Here's the drawing with two shaded views (mm, measured from the low corner). I have some questions. Round coordinates to 2 decimals unless told otherwise and drop trailing zeros. Loops run counter-clockwise (first coordinate to the right, second up) from the corner with the lowest first, then second, coordinate; pieces in that order, holes last. Notation, with made-up numbers: (7.5, 19) -> (37.5, 19) arc R24 ccw to (37.5, 58) -> close; hole circle Ø1 at (44.5, -14.75). An arc over 180 degrees is marked (long way). Write item = value, one per line.
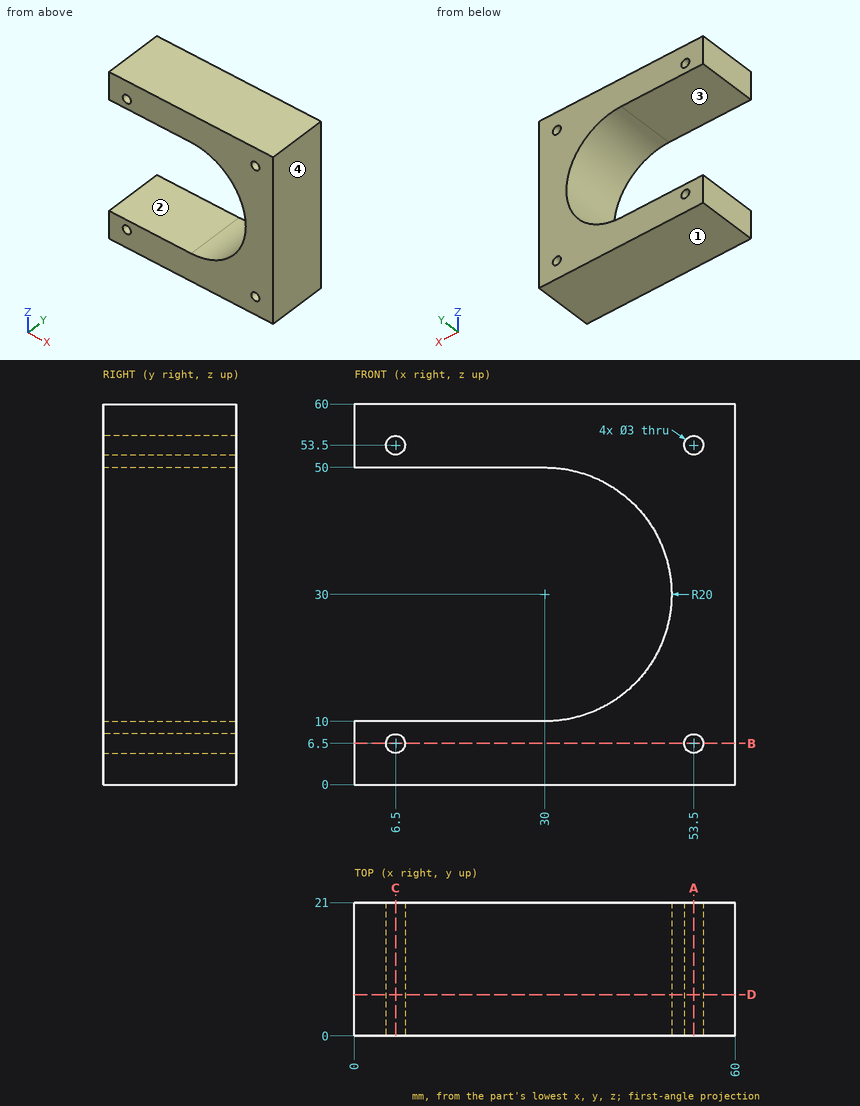
1. I need wall thicknesses on line 1 (X direction, y = 7, z = 53.5); line 2 (Z direction, x = 6.5, y = 15). Which ranges of each line are inside material? Lowest first, please. Write a range as [from, to].
Entries:
line_1 = [0, 5], [8, 52], [55, 60]
line_2 = [0, 5], [8, 10], [50, 52], [55, 60]
2. Suppose I cut it at C-C, the plane x = 6.5. List the corners of the cut face in (y, z) for me.
Entries:
outline = (0, 0) -> (21, 0) -> (21, 5) -> (0, 5) -> close; (0, 8) -> (21, 8) -> (21, 10) -> (0, 10) -> close; (0, 50) -> (21, 50) -> (21, 52) -> (0, 52) -> close; (0, 55) -> (21, 55) -> (21, 60) -> (0, 60) -> close
3. Suppose I cut it at B-B, the plane z = 6.5. List the corners of the cut face in (x, y) for me.
Entries:
outline = (0, 0) -> (5, 0) -> (5, 21) -> (0, 21) -> close; (8, 0) -> (52, 0) -> (52, 21) -> (8, 21) -> close; (55, 0) -> (60, 0) -> (60, 21) -> (55, 21) -> close
4. I'm going to push flat-ended pins straight in: pin 1 (2.5 mm diameter, centred on x = 6.5, z = 53.5, fed in from +Y); pin 2 (8 mm diameter, centred on y = 8, z = 25.5, fed in from -X); pin 3 (4 mm diameter, centred on y = 12.5, z = 31.5, fed in from -X). Where does each tip first touch, or does it pass through?
Entries:
pin_1 = through
pin_2 = 48.1
pin_3 = 49.69
5. Suppose I cut it at A-A, the plane x = 53.5. List the corners of the cut face in (y, z) for me, and give its area (3 significant figures).
Entries:
outline = (0, 0) -> (21, 0) -> (21, 5) -> (0, 5) -> close; (0, 8) -> (21, 8) -> (21, 52) -> (0, 52) -> close; (0, 55) -> (21, 55) -> (21, 60) -> (0, 60) -> close
area = 1,130 mm²
6. Suppose I cut it at D-D, the plane y = 6.5. List the corners of the cut face in (x, z) for me, and give its area (3 significant figures).
Entries:
outline = (0, 0) -> (60, 0) -> (60, 60) -> (0, 60) -> (0, 50) -> (30, 50) arc R20 cw to (30, 10) -> (0, 10) -> close; hole circle Ø3 at (6.5, 6.5); hole circle Ø3 at (6.5, 53.5); hole circle Ø3 at (53.5, 6.5); hole circle Ø3 at (53.5, 53.5)
area = 1,740 mm²
7. We'd pull the mould along Z, two halves only. Please class the marked faces 1, 2, 3 and 4: released by +Z, released by -Z, zero draft, split by the parting line, or undercut.
Entries:
face_1 = released by -Z
face_2 = undercut
face_3 = undercut
face_4 = zero draft
